Check sheet for the modelled part. Datum: model origin and axes. Units: mm. Round coordinates to 2 decimals unless told otherwise and drop trailing zeros. Loops run counter-clockwise (first coordinate to the right, second up) from the corner with the lowest first, then second, coordinate; pieces in that order, holes last. Notation, with made-up numbers: (47.5, 16.25) - (97.5, 16.25) arc R28 ccw to (97.5, 54.25) - close; hole circle Ø4 at (76.25, 32). An arc over 180 degrees is marked (long way). Return JSON: item names as keys, results as strings.
from build123d import *

# Parameters (mm, degrees)
SKETCH_W        = 100
SKETCH_H        = 100
PAD_DEPTH       = 5
POCKET_DEPTH    = 100
POCKET001_DEPTH = 100


with BuildPart() as part:
    # Sketch → Pad (new body)
    with BuildSketch(Plane.XY):
        Rectangle(SKETCH_W, SKETCH_H)
    extrude(amount=PAD_DEPTH)

    # Sketch001 (on Face1 of Pad) → Pocket (cut)
    with BuildSketch(Plane.XZ.offset(50)):
        Polygon((-50, 0), (-47.928932, 5), (-50, 5), align=None)
    extrude(amount=-POCKET_DEPTH, mode=Mode.SUBTRACT)

    # Sketch002 (on Face1 of Pocket) → Pocket001 (cut)
    with BuildSketch(Plane.XZ.offset(50)):
        Polygon((50, 0), (47.928932, 5), (50, 5), align=None)
    extrude(amount=-POCKET001_DEPTH, mode=Mode.SUBTRACT)


solid = part.part
Q1. Depth check by flat-ended pin: P1, Ø1.5, axis at y = -14.5, z = 3, coming from the +X side. Enter the tip coordinate at first touch or a pass-through.
Answer key:
{"P1": "stops at x = 49.07"}
Q2. Sectioned sample at B-B (z = 2.5). Enter the section's corners in (x, y), plus the area to 3 significant figures.
Answer key:
{"outline": "(-48.96, -50) - (48.96, -50) - (48.96, 50) - (-48.96, 50) - close", "area": "9,790 mm²"}
Q3. Scan lines: probe 1 along X at (y, z) = (21, 2.1); probe 2 along X at (y, z) = (6, 2.3). Record each from-to range of solid material in increasing order. Write a range as [from, to].
Answer key:
{"probe 1": "x = [-49.13, 49.13]", "probe 2": "x = [-49.05, 49.05]"}
Q4. Sectioned sample at A-A (y = 21). Enter the section's corners in (x, z), plus the area to 3 significant figures.
Answer key:
{"outline": "(-50, 0) - (50, 0) - (47.93, 5) - (-47.93, 5) - close", "area": "490 mm²"}
